```python
from build123d import *


with BuildPart() as part:
    # Sketch1 → Revolve1 (revolve)
    with BuildSketch(Plane.XY):
        with BuildLine():
            Line((0, 23.55), (3, 23.55))
            Line((3, 23.55), (3, 17.9))
            Line((3, 17.9), (2, 17.9))
            Line((2, 17.9), (2, 14.6))
            Line((2, 14.6), (3.4, 14.6))
            Line((3.4, 14.6), (3.4, 8.7))
            Line((3.4, 8.7), (4.85, 8.7))
            Line((4.85, 8.7), (4.85, 6.845))
            ThreePointArc((4.85, 6.845), (4.573215908, 6.176784092), (3.905, 5.9))
            Line((3.905, 5.9), (3.905, 0))
            Line((3.905, 0), (0, 0))
            Line((0, 0), (0, 23.55))
        make_face()
    revolve(axis=Axis((0, 0, 0), (0, 1, 0)))


solid = part.part
```
Model file for the job. Use its own axes, mm. A direction names the side the tool comes from. Round coordinates to 2 decimals unless told otherwise and drop trailing zeros. Write each loop counter-clockwise with the first axis right and the second up, starting at its lowest first coordinate (ties: lowest second). Pieces come first, ordered by that corner, then holes. Notation, with made-up numbers: (66.5, 1.5) - (85.5, 1.5) arc R22 ccw to (85.5, 20.5) - close; hole circle Ø6 at (71, 5). An arc over 180 degrees is marked (long way). Use CSV: the item, a comma, the result in double quotes. Start each with the question number.
Item 1: Band-saw the part on A-A (z = 0). Write the cut outline in (x, y) (3 decimals), and give its area (3 significant figures).
Item 2: Tool access for faces 4 (the face through (-0.74, 11.61, 3.32)), 5 (the face through (0, 0, 0)), 6 (the face through (0, 16, 2)), 7 (the face through (-0.85, 2.91, 3.81)): list every direction of +Z, -Z, +X, -X, +Y, -Y with a clear straight run to the whole face (end or side of a thin tool).
Item 3: Pin check, flat tips, straight feed: P1, Ø3, axis at x = -2, y = 18.5, coming from the +Z side; P2, Ø1.5, axis at x = -1.5, y = 11, coming from the -Z side; P3, Ø5, axis at y = 20.5, z = 0, coming from the +X side. Stop position of each tip, or through.
Item 4: Drill centre lines: L1, parallel to Y at x = 0.5, z = -3.5; L2, parallel to Y at x = 1, z = -3; L3, parallel to X at y = 9.75, z = 2.75. Where is each one in solid material? Low to high. Write a range as [from, to].
Item 5: Band-saw the part on D-D (y = 22). Write the cut outline in (x, z), and give its area (3 significant figures).
Item 6: Two-plate mould, pull along Y, no slides. Class faces 1 (the face through (-3, 21, 0)), 2 (the face through (0, 23.55, 0)), 3 (the face through (1, 17.9, 2)): released by +Y, released by -Y, zero draft, split by the parting line, or undercut.
Item 7: Band-saw the part on C-C (y = 16.5). Write the cut outline in (x, z).
Item 8: Band-saw the part on B-B (x = 0). Write the cut outline in (y, z) (3 decimals).
Checked values:
1,outline,"(-4.85, 6.845) arc R0.945 ccw to (-3.905, 5.9) - (-3.905, 0) - (3.905, 0) - (3.905, 5.9) arc R0.945 ccw to (4.85, 6.845) - (4.85, 8.7) - (3.4, 8.7) - (3.4, 14.6) - (2, 14.6) - (2, 17.9) - (3, 17.9) - (3, 23.55) - (-3, 23.55) - (-3, 17.9) - (-2, 17.9) - (-2, 14.6) - (-3.4, 14.6) - (-3.4, 8.7) - (-4.85, 8.7) - close"
1,area,"160 mm²"
2,face 4,"+Y"
2,face 5,"+Z, -Z, +X, -X, -Y"
2,face 6,"none"
2,face 7,"-Y"
3,P1,"stops at z = 2.96"
3,P2,"stops at z = -3.32"
3,P3,"stops at x = 3"
4,L1,"y = [0, 8.7]"
4,L2,"y = [0, 14.6]"
4,L3,"x = [-2, 2]"
5,outline,"circle Ø6 at (0, 0)"
5,area,"28.3 mm²"
6,face 1,"zero draft"
6,face 2,"released by +Y"
6,face 3,"undercut"
7,outline,"circle Ø4 at (0, 0)"
8,outline,"(0, -3.905) - (5.9, -3.905) arc R0.945 ccw to (6.845, -4.85) - (8.7, -4.85) - (8.7, -3.4) - (14.6, -3.4) - (14.6, -2) - (17.9, -2) - (17.9, -3) - (23.55, -3) - (23.55, 3) - (17.9, 3) - (17.9, 2) - (14.6, 2) - (14.6, 3.4) - (8.7, 3.4) - (8.7, 4.85) - (6.845, 4.85) arc R0.945 ccw to (5.9, 3.905) - (0, 3.905) - close"
